CAD build for the part. Positions are in the model's coordinates, mm. A direction names the side the tool comes from. Coordinates: 2 decimals unless noted, no trailing zeros. Order: outer loops, then holes, each group sorted by start corner. A loop starts at its lowest first (then second) coordinate and runs counter-clockwise, first axis right, second up. Notation, with made-up numbers: M 47.5,54 L 58.5,54 A24 ccw 58.5,67 Z; hole C 47.25,19 d7. An arc over 180 degrees is marked long. Write item = value, one per line.
from build123d import *

# Parameters (mm, degrees)
F0_W      = 127
F0_H      = 63.5
F1_DEPTH  = 38.1
F2_W      = 12.7
F2_H      = 9.525
F3_DEPTH  = 127
F4_R      = 9.525
F5_DEPTH  = 25.4
F5_FACE_R = 9.525
F6_DEPTH  = 63.78913
F7_R      = 9.525
F8_DEPTH  = 127.28539


with BuildPart() as f1:
    # F0 (on Top) → F1 (new body)
    with BuildSketch(Plane.XY):
        with Locations((63.5, -31.75)):
            Rectangle(F0_W, F0_H)
    extrude(amount=F1_DEPTH)

    # F2 (on face) → F3 (cut)
    with BuildSketch(Plane.YZ.offset(127)):
        with Locations((-57.15, 33.3375)):
            Rectangle(F2_W, F2_H)
        with Locations((-57.15, 4.7625)):
            Rectangle(F2_W, F2_H)
    extrude(amount=-F3_DEPTH, mode=Mode.SUBTRACT)

    # F4 (on face) → F5 (join)
    with BuildSketch(Plane.XY.offset(38.1)):
        with Locations((31.75, -18.866556)):
            Circle(F4_R)
        with Locations((95.25, -18.669)):
            Circle(F4_R)
    extrude(amount=F5_DEPTH)

    # F5_face (on face) → F6 (cut)
    with BuildSketch(Plane(origin=(31.75, -18.866556, 63.5), x_dir=(1, 0, 0), z_dir=(0, 0, 1))):
        Circle(F5_FACE_R)
        with Locations((63.5, 0.197556)):
            Circle(F5_FACE_R)
    extrude(amount=-F6_DEPTH, mode=Mode.SUBTRACT)

    # F7 (on face) → F8 (cut)
    with BuildSketch(Plane.YZ.offset(127)):
        with Locations((-25.4, 19.05)):
            Circle(F7_R)
    extrude(amount=-F8_DEPTH, mode=Mode.SUBTRACT)


solid = f1.part
(1) Slice it at B-B, the plane y = -25.5. Write the cut outline in (x, z).
Evaluation:
outline = M 0,0 L 24.91,0 L 24.91,9.53 L 0,9.53 Z; M 0,28.57 L 24.91,28.57 L 24.91,38.1 L 0,38.1 Z; M 38.59,0 L 88.61,0 L 88.61,9.53 L 38.59,9.53 Z; M 38.59,28.57 L 88.61,28.57 L 88.61,38.1 L 38.59,38.1 Z; M 101.89,0 L 127,0 L 127,9.53 L 101.89,9.53 Z; M 101.89,28.57 L 127,28.57 L 127,38.1 L 101.89,38.1 Z
(2) Wall check: line 1 (Z direction, x = 69, y = -25); line 2 (Y direction, x = 59, z = 19); line 3 (Y direction, x = 62.5, z = 8). Give the ranges that are in metal, low to high. Write a range as from..to.
Evaluation:
line_1 = 0..9.53, 28.57..38.1
line_2 = -63.5..-34.92, -15.88..0
line_3 = -50.8..0
(3) Pin check, flat tips, straight feed: pin 1 Ø4 at (x, y) = (76, -60) entering from +Z (3 decimals); pin 2 Ø5 at (x, z) = (87.5, 5) entering from -Y; pin 3 Ø4 at (x, y) = (60, -58.5) entering from -Z (3 decimals). Stop position of each tip, or through.
Evaluation:
pin_1 = 28.575
pin_2 = -50.8
pin_3 = 9.525
(4) Slice it at A-A, the plane x = 31.75. Write the cut outline in (y, z) (3 decimals).
Evaluation:
outline = M -63.5,9.525 L -50.8,9.525 L -50.8,0 L -28.392,0 L -28.392,10.007 A9.525 cw -28.392,28.093 L -28.392,38.1 L -50.8,38.1 L -50.8,28.575 L -63.5,28.575 Z; M -9.342,0 L 0,0 L 0,38.1 L -9.342,38.1 Z
(5) Slice it at C-C, the plane z = 19.05. Write the cut outline in (x, y) (3 decimals), then the cut area to 3 significant figures.
Evaluation:
outline = M 0,-63.5 L 127,-63.5 L 127,-34.925 L 0,-34.925 Z; M 0,-15.875 L 22.707,-15.875 A9.525 cw 40.793,-15.875 L 86.144,-15.875 A9.525 cw 104.356,-15.875 L 127,-15.875 L 127,0 L 0,0 Z
area = 5,470 mm²
(6) Pull direction X, two halves, no side cores. Call faces 4 (the face through (0, -32, 27)), 5 (the face through (30.51, -9.423, 19.317)), 6 (the face through (63, -25, 38.1)): +X half, -X half, draft (parallel to the pull), parting line (faces both ways), or undercut.
Evaluation:
face_4 = -X half
face_5 = undercut
face_6 = draft
(7) Tool access for faces 1 (the face through (64.389, -34.916, 19.469)), 2 (the face through (64, -50.8, 5)), 3 (the face through (64, -50.8, 33)): list every direction of +Z, -Z, +X, -X, +Y, -Y with a clear straight run to the whole face (end or side of a thin tool).
Evaluation:
face_1 = +X, -X
face_2 = -Z, +X, -X, -Y
face_3 = +Z, +X, -X, -Y
(8) Slice it at D-D, the plane x = 119. Write the cut outline in (y, z) (3 decimals).
Evaluation:
outline = M -63.5,9.525 L -50.8,9.525 L -50.8,0 L 0,0 L 0,38.1 L -50.8,38.1 L -50.8,28.575 L -63.5,28.575 Z; hole C -25.4,19.05 d19.05
